from build123d import *

# Parameters (mm, degrees)
SKETCH_1_W          = 120
SKETCH_1_H          = 27
SKETCH_1_R          = 2
SKETCH_1_R_2        = 1.5
EXTRUDE_1_DEPTH     = 4
CUT_EXTRUDE_1_DEPTH = 10
FILLET_1_R          = 2


with BuildPart() as part:
    # 草图1 → 凸台-拉伸1 (new body)
    with BuildSketch(Plane.XY):
        Rectangle(SKETCH_1_W, SKETCH_1_H)
        with Locations((56, 5.5)):
            Circle(SKETCH_1_R, mode=Mode.SUBTRACT)
        with Locations((56, -9.5)):
            Circle(SKETCH_1_R, mode=Mode.SUBTRACT)
        with Locations((25, -10.5)):
            Circle(SKETCH_1_R_2, mode=Mode.SUBTRACT)
        with Locations((5, -10.5)):
            Circle(SKETCH_1_R_2, mode=Mode.SUBTRACT)
    extrude(amount=EXTRUDE_1_DEPTH)

    # 草图2 → 切除-拉伸1 (cut)
    with BuildSketch(Plane(origin=(0, 0, 0), x_dir=(-1, 0, 0), z_dir=(0, 0, -1))):
        Polygon((60, -8.5), (-12, 13.5), (60, 13.5), align=None)
    extrude(amount=-CUT_EXTRUDE_1_DEPTH, mode=Mode.SUBTRACT)

    # 圆角1
    fillet_1_edges = [part.edges().sort_by_distance(p)[0] for p in [
        (-60, -8.5, 2),
        (12, 13.5, 2),
        (60, -13.5, 2),
        (-60, -13.5, 2),
        (60, 13.5, 2),
    ]]
    fillet(fillet_1_edges, radius=FILLET_1_R)


solid = part.part
Geometry: final body of the model. Coordinates: model frame, mm. Coordinates: 2 decimals unless noted, no trailing zeros. Write each loop counter-clockwise with the first axis right and the second up, starting at its lowest first coordinate (ties: lowest second). Pieces come first, ordered by that corner, then holes. Notation, with made-up numbers: (-3.5, 88) - (2.5, 88) arc R32 ccw to (2.5, 124) - close; hole circle Ø2 at (81, -37). An arc over 180 degrees is marked (long way). Return JSON: item names as keys, results as strings.
Item 1: Section query A-A (x = 25). Output: boundary loops of the cut face in (y, z).
Completed:
{"outline": "(-13.5, 0) - (-12, 0) - (-12, 4) - (-13.5, 4) - close; (-9, 0) - (13.5, 0) - (13.5, 4) - (-9, 4) - close"}
Item 2: Line query: L1, parallel to Y at x = 12, z = 3.75; L2, parallel to Y at x = 8, z = 2.8. Output: solid intervals per line, ascending.
Completed:
{"L1": "y = -13.5 to 13.48", "L2": "y = -13.5 to 12.28"}
Item 3: Section query D-D (y = 5.5). Output: boundary loops of the cut face in (x, z).
Completed:
{"outline": "(-14.18, 0) - (54, 0) - (54, 4) - (-14.18, 4) - close; (58, 0) - (60, 0) - (60, 4) - (58, 4) - close"}
Item 4: Pull-direction query (X, two-part tool) for faces 1 (the face through (5.69, -11.83, 1.97)), 2 (the face through (-23.93, 2.52, 1.97)), 3 (the face through (-1, -13.5, 2)), 4 (the face through (60, 0, 2)); classes: +X half, -X half, draft (parallel to the pull), parting line (faces both ways), or undercut.
Completed:
{"face 1": "undercut", "face 2": "-X half", "face 3": "draft", "face 4": "+X half"}
Item 5: Section query B-B (z = 2.6). Output: boundary loops of the cut face in (x, y).
Completed:
{"outline": "(-60, -11.5) arc R2 ccw to (-58, -13.5) - (58, -13.5) arc R2 ccw to (60, -11.5) - (60, 11.5) arc R2 ccw to (58, 13.5) - (12.3, 13.5) arc R2 ccw to (11.71, 13.41) - (-58.58, -8.07) arc R2 ccw to (-60, -9.98) - close; hole circle Ø3 at (5, -10.5); hole circle Ø3 at (25, -10.5); hole circle Ø4 at (56, -9.5); hole circle Ø4 at (56, 5.5)"}
Item 6: Section query C-C (x = 56). Output: boundary loops of the cut face in (y, z), and give its area (3 significant figures).
Completed:
{"outline": "(-13.5, 0) - (-11.5, 0) - (-11.5, 4) - (-13.5, 4) - close; (-7.5, 0) - (3.5, 0) - (3.5, 4) - (-7.5, 4) - close; (7.5, 0) - (13.5, 0) - (13.5, 4) - (7.5, 4) - close", "area": "76.0 mm2"}
Item 7: Pin query (flat end, axial travel): pin 1 Ø3 at (x, y) = (56, -9.5) entering from +Z. Return the tip coordinate at first contact, or that it passes through.
Completed:
{"pin 1": "passes through"}
